Design review of the part built by this model. Coordinates are the model's own, in mm. Face numbers are marked on the shaded views. A direction names the side the tool comes from. Give positions to 0.01 mm unless a question says otherwise; leave off trailing zeros. Write each loop counter-clockwise with the first axis right and the second up, starting at its lowest first coordinate (ties: lowest second). Pieces come first, ordered by that corner, then holes. Notation, with made-up numbers: M 17.25,64 L 23.25,64 A9 cw 23.25,68 Z; hole C 9.25,48 d5. An arc over 180 degrees is marked long. Use one line per item in the form item = value. Start each with the question number.
from build123d import *

# Parameters (mm, degrees)
SKETCH1_W           = 17
SKETCH1_H           = 12
SKETCH1_R           = 3
BOSS_EXTRUDE1_DEPTH = 2
SKETCH2_W           = 17
SKETCH2_H           = 12
SKETCH2_W_2         = 14
SKETCH2_H_2         = 9
BOSS_EXTRUDE2_DEPTH = 23
CHAMFER1_SIZE       = 0.5


with BuildPart() as part:
    # Sketch1 → Boss-Extrude1 (new body)
    with BuildSketch(Plane(origin=(0, 0, 0), x_dir=(1, 0, 0), z_dir=(0, 1, 0))):
        Rectangle(SKETCH1_W, SKETCH1_H)
        with Locations(Location((0, 0, 0), (0, 0, 270))):
            Circle(SKETCH1_R, mode=Mode.SUBTRACT)
    extrude(amount=BOSS_EXTRUDE1_DEPTH)

    # Sketch2 → Boss-Extrude2 (add)
    with BuildSketch(Plane(origin=(0, 0, 0), x_dir=(1, 0, 0), z_dir=(0, 1, 0))):
        Rectangle(SKETCH2_W, SKETCH2_H)
        Rectangle(SKETCH2_W_2, SKETCH2_H_2, mode=Mode.SUBTRACT)
    extrude(amount=-BOSS_EXTRUDE2_DEPTH)

    # Chamfer1
    chamfer1_edges = [part.edges().sort_by_distance(p)[0] for p in [
        (0, 2, -3),
    ]]
    chamfer(chamfer1_edges, length=CHAMFER1_SIZE)


solid = part.part
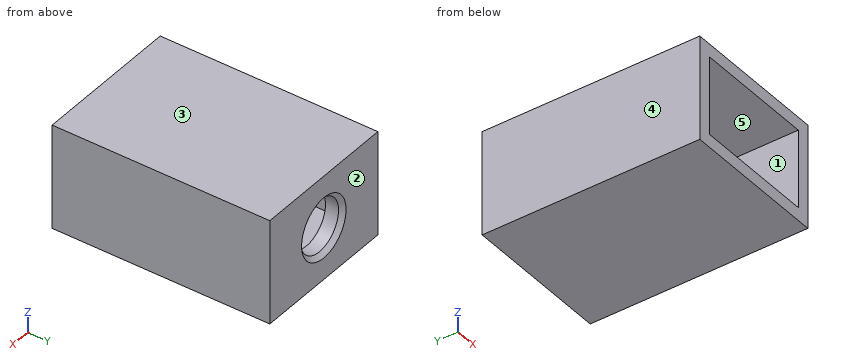
1. We need section C-C (x = 0). State the section outline as (y, z) points, and give its area (4 significant figures).
2. To check wall thickness, follow L1, parallel to Z at x = -2, y = -16.75; L2, parallel to X at y = -8, z = 3.5; L3, parallel to X at y = 1, z = 0. State the ranges of each line that lie inside material, in increasing order.
3. Clearance check with flat-ended pins moving along their axes: pin 1 Ø2.5 at (x, z) = (-0.5, 2) entering from -Y; pin 2 Ø5 at (x, z) = (0, 0) entering from -Y. State where each tip first meets the part, or that it passes through.
4. We need section A-A (z = 0). State the section outline as (x, y) points, and give its area (4 significant figures).
5. We need section D-D (x = -4.75). State the section outline as (y, z) points, and give its area (3 significant figures).
6. We need section B-B (y = -13.25). State the section outline as (x, z) points.
7. For the marked faces 4 and 5, list the 3-axis set-ups (+Z, -Z, +X, -X, +Y, -Y) from which the entire face can be reached by the end or side of a thin tool; tool diameter is ignored.
8. Draft analysis for pull direction Z (two halves, no side actions). For the marked faces 1, 2 and 3, state which applies: pulls with the +Z half, pulls with the -Z half, needs draft (parallel to the pull), parting line crosses it, or undercut.
Answer block:
q1.outline = M -23,-6 L 2,-6 L 2,-3.5 L 1.5,-3 L 0,-3 L 0,-4.5 L -23,-4.5 Z; M -23,4.5 L 0,4.5 L 0,3 L 1.5,3 L 2,3.5 L 2,6 L -23,6 Z
q1.area = 80.75 mm^2
q2.L1 = -6 to -4.5, 4.5 to 6
q2.L2 = -8.5 to -7, 7 to 8.5
q2.L3 = -8.5 to -3, 3 to 8.5
q3.pin_1 = 0
q3.pin_2 = through
q4.outline = M -8.5,-23 L -7,-23 L -7,0 L -3,0 L -3,1.5 L -3.5,2 L -8.5,2 Z; M 3,0 L 7,0 L 7,-23 L 8.5,-23 L 8.5,2 L 3.5,2 L 3,1.5 Z
q4.area = 90.75 mm^2
q5.outline = M -23,-6 L 2,-6 L 2,6 L -23,6 L -23,4.5 L 0,4.5 L 0,-4.5 L -23,-4.5 Z
q5.area = 93.0 mm^2
q6.outline = M -8.5,-6 L 8.5,-6 L 8.5,6 L -8.5,6 Z; hole M -7,-4.5 L 7,-4.5 L 7,4.5 L -7,4.5 Z
q7.face_4 = +Z, -Z, -X, +Y, -Y
q7.face_5 = -Y
q8.face_1 = undercut
q8.face_2 = needs draft
q8.face_3 = pulls with the +Z half
